from build123d import *

# Parameters (mm, degrees)
SKETCH1_R           = 3.175
BOSS_EXTRUDE1_DEPTH = 60.198
SKETCH2_R           = 2.667
BOSS_EXTRUDE2_DEPTH = 1.016
SKETCH3_R           = 3.175
BOSS_EXTRUDE3_DEPTH = 1.524
BOSS_EXTRUDE4_START = 1.016
SKETCH4_R           = 2.667
BOSS_EXTRUDE4_DEPTH = 1.016
BOSS_EXTRUDE5_START = 1.524
SKETCH7_R           = 3.175
BOSS_EXTRUDE5_DEPTH = 1.524


with BuildPart() as part:
    # Sketch1 → Boss-Extrude1 (new body)
    with BuildSketch(Plane(origin=(0, 0, 0), x_dir=(1, 0, 0), z_dir=(0, 1, 0))):
        with Locations(Location((0, 0, 0), (0, 0, 90))):
            Circle(SKETCH1_R)
    extrude(amount=BOSS_EXTRUDE1_DEPTH)

    # Sketch2 → Boss-Extrude2 (add)
    with BuildSketch(Plane(origin=(0, 60.198, 0), x_dir=(1, 0, 0), z_dir=(0, 1, 0))):
        with Locations(Location((0, 0, 0), (0, 0, 270))):
            Circle(SKETCH2_R)
    extrude(amount=BOSS_EXTRUDE2_DEPTH)

    # Sketch3 → Boss-Extrude3 (add)
    with BuildSketch(Plane(origin=(0, 61.214, 0), x_dir=(1, 0, 0), z_dir=(0, 1, 0))):
        with Locations(Location((0, 0, 0), (0, 0, 90))):
            Circle(SKETCH3_R)
    extrude(amount=BOSS_EXTRUDE3_DEPTH)

    # Sketch4 → Boss-Extrude4 (add)
    with BuildSketch(Plane.XZ.offset(BOSS_EXTRUDE4_START)):
        with Locations(Location((0, 0, 0), (0, 0, 90))):
            Circle(SKETCH4_R)
    extrude(amount=-BOSS_EXTRUDE4_DEPTH)

    # Sketch7 → Boss-Extrude5 (add)
    with BuildSketch(Plane(origin=(0, -1.016, 0), x_dir=(-1, 0, 0), z_dir=(0, -1, 0)).offset(BOSS_EXTRUDE5_START)):
        with Locations(Location((0, 0, 0), (0, 0, 90))):
            Circle(SKETCH7_R)
    extrude(amount=-BOSS_EXTRUDE5_DEPTH)


solid = part.part
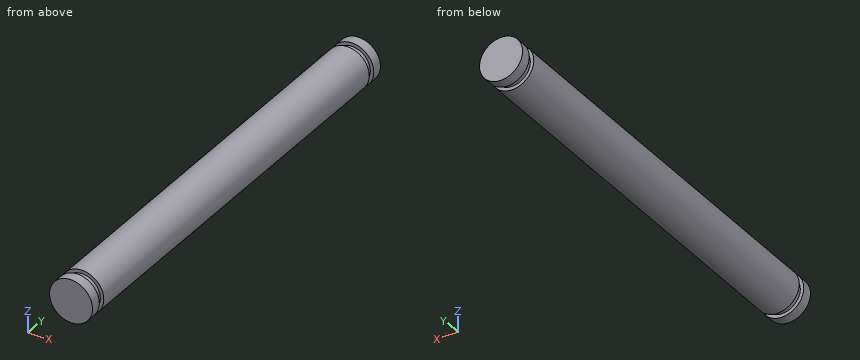
The listing builds one solid part. Answer for the finished solid, in the listing's coordinates (mm). Round coordinates to 2 decimals unless told otherwise and drop trailing zeros. Loops run counter-clockwise (first coordinate to the right, second up) from the corner with the lowest first, then second, coordinate; pieces in that order, holes last. Notation, with made-up numbers: M 5,37 L 37,37 A5 cw 37,44 Z; hole C -34.5,40 d1. An arc over 180 degrees is marked long. Return JSON: item names as keys, results as strings.
Q1. Each of these flat-tipped pins is pushed along its axis until it touches: pin 1 Ø1.5 at (y, z) = (17, 2) entering from -X; pin 2 Ø2 at (y, z) = (5.5, -2) entering from -X. Where does it stop, or does it pass through?
Results list:
{"pin 1": "stops at x = -2.92", "pin 2": "stops at x = -3.01"}
Q2. Find section C-C, the plane y = 19.5. Determine the outline of the cut face in (x, z) (3 decimals).
Results list:
{"outline": "C 0,0 d6.35"}
Q3. Find section A-A, the plane z = -1.5. Determine the outline of the cut face in (x, y), plus the area to 3 significant figures.
Results list:
{"outline": "M -2.8,-2.54 L 2.8,-2.54 L 2.8,-1.02 L 2.21,-1.02 L 2.21,0 L 2.8,0 L 2.8,60.2 L 2.21,60.2 L 2.21,61.21 L 2.8,61.21 L 2.8,62.74 L -2.8,62.74 L -2.8,61.21 L -2.21,61.21 L -2.21,60.2 L -2.8,60.2 L -2.8,0 L -2.21,0 L -2.21,-1.02 L -2.8,-1.02 Z", "area": "363 mm2"}
Q4. Find the intervals of material crossed by line 1 along Y through (x, z) = (2.25, -2); line 2 along X through (y, z) = (42, -0.25), in increasing order. Write a range as from..to.
Results list:
{"line 1": "y = -2.54..-1.02, 0..60.2, 61.21..62.74", "line 2": "x = -3.17..3.17"}
Q5. Find section B-B, the plane x = 0.75. Determine the outline of the cut face in (y, z).
Results list:
{"outline": "M -2.54,-3.09 L -1.02,-3.09 L -1.02,-2.56 L 0,-2.56 L 0,-3.09 L 60.2,-3.09 L 60.2,-2.56 L 61.21,-2.56 L 61.21,-3.09 L 62.74,-3.09 L 62.74,3.09 L 61.21,3.09 L 61.21,2.56 L 60.2,2.56 L 60.2,3.09 L 0,3.09 L 0,2.56 L -1.02,2.56 L -1.02,3.09 L -2.54,3.09 Z"}
